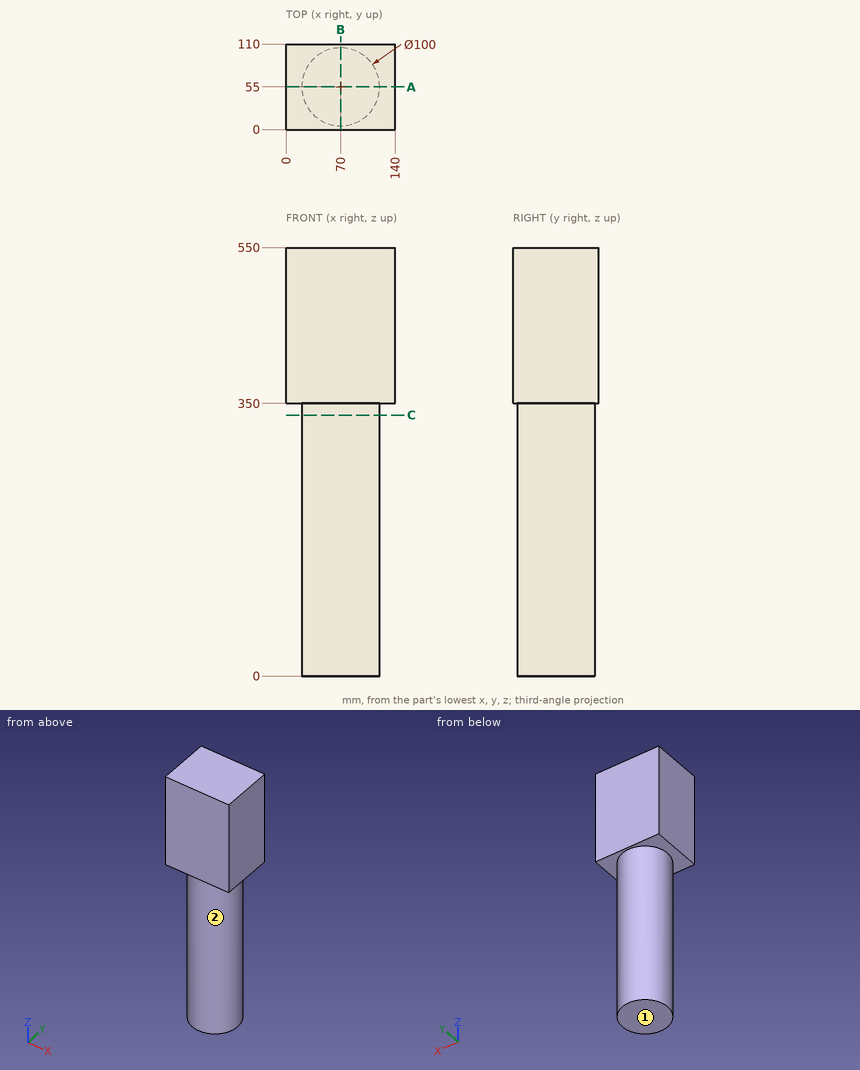
Geometry: see drawing. Coordinates: mm, zero at the bounding-box minimum. A direction names the side the tool comes from. Coordinates: 2 decimals unless noted, no trailing zeros. Loops run counter-clockwise (first coordinate to the right, second up) from the corner with the lowest first, then second, coordinate; pieces in that order, holes last. Notation, with made-up numbers: M -11,71.5 L -3,71.5 A18 ccw -3,84.5 Z; hole C 55,-6.5 d2. An arc over 180 degrees is marked long. Answer in a Markdown table with one row per item.
Q1. Ray query, probe 1 along Z at (x, y) = (120, 22.5); probe 2 along X at (y, z) = (51, 230.5); probe 3 along Y at (x, z) = (30, 202). Return the intervals inside material, ascending. Write a range as from..to.
Answers below:
| item | result |
|---|---|
| probe 1 | z = 350..550 |
| probe 2 | x = 20.16..119.84 |
| probe 3 | y = 25..85 |
Q2. Section C-C on z = 335. Return the cut outline in (x, y), plus the area to 3 significant figures.
Answers below:
| item | result |
|---|---|
| outline | C 70,55 d100 |
| area | 7,850 mm^2 |
Q3. First-contact query: pin 1 (12 mm diameter, centred on x = 121.5, z = 390.5, fed in from -Y); pin 2 (6 mm diameter, centred on x = 106.5, z = 248, fed in from -Y); pin 3 (12 mm diameter, centred on x = 26.5, y = 15.5, fed in from -Z). Flat tips, straight axial feed; report the tip coordinate or a pass-through.
Answers below:
| item | result |
|---|---|
| pin 1 | stops at y = 0 |
| pin 2 | stops at y = 17.88 |
| pin 3 | stops at z = 350 |
Q4. Section B-B on x = 70. Return the cut outline in (y, z).
Answers below:
| item | result |
|---|---|
| outline | M 0,350 L 5,350 L 5,0 L 105,0 L 105,350 L 110,350 L 110,550 L 0,550 Z |
Q5. Set-up query: the marked faces 1 and 2. Return all of +Z, -Z, +X, -X, +Y, -Y with unobstructed straight access to the full face (end or side cutting, diameter ignored); none if empty.
Answers below:
| item | result |
|---|---|
| face 1 | -Z, +X, -X, +Y, -Y |
| face 2 | -Z |
Q6. Section A-A on y = 55. Return the cut outline in (x, z).
Answers below:
| item | result |
|---|---|
| outline | M 0,350 L 20,350 L 20,0 L 120,0 L 120,350 L 140,350 L 140,550 L 0,550 Z |
